Can you work these out from the model? Positions are in its coordinate system, mm. Face numbers are marked on the shaded views. A direction names the side the tool comes from. Round coordinates to 2 decimals unless told otherwise and drop trailing zeros. Loops run counter-clockwise (first coordinate to the right, second up) from the corner with the lowest first, then second, coordinate; pieces in that order, holes last. Notation, with made-up numbers: (-16.5, 27) -> (-3.5, 27) arc R22 ccw to (-3.5, 37) -> close; hole circle Ø8 at (9, 66). An arc over 180 degrees is marked (long way). Write each question's results on one line, items separated by ' | '.
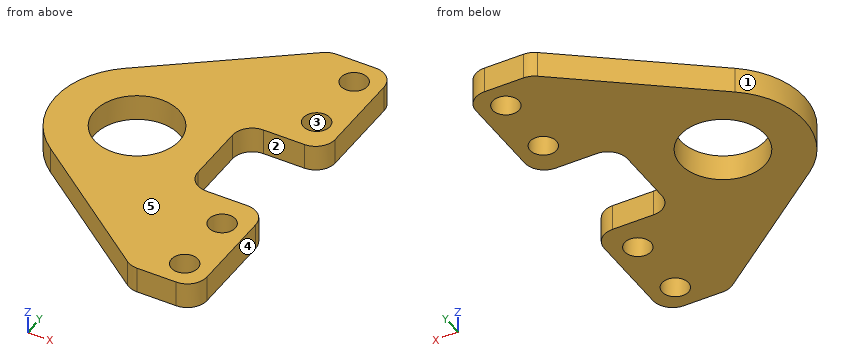
from build123d import *

# Parameters (mm, degrees)
SKETCH_1_R          = 6.5
SKETCH_1_R_2        = 2.025
EXTRUDE_1_DEPTH     = 2
SKETCH_2_W          = 12.3
SKETCH_2_H          = 15.2
CUT_EXTRUDE_1_DEPTH = 10
FILLET_1_R          = 3


with BuildPart() as part:
    # 草图1 → 凸台-拉伸1 (new, symmetric)
    with BuildSketch(Plane.XY):
        with BuildLine():
            Line((-7.572670512, 9.945082268), (14.3, 26.6))
            Line((14.3, 26.6), (24.3, 26.6))
            Line((24.3, 26.6), (24.3, -26.6))
            Line((24.3, -26.6), (14.3, -26.6))
            Line((14.3, -26.6), (-7.572670512, -9.945082268))
            ThreePointArc((-7.572670512, -9.945082268), (-12.5, 0), (-7.572670512, 9.945082268))
        make_face()
        Circle(SKETCH_1_R, mode=Mode.SUBTRACT)
        with Locations((20.3, 22.6)):
            Circle(SKETCH_1_R_2, mode=Mode.SUBTRACT)
        with Locations((20.3, 12.6)):
            Circle(SKETCH_1_R_2, mode=Mode.SUBTRACT)
        with Locations((20.3, -12.6)):
            Circle(SKETCH_1_R_2, mode=Mode.SUBTRACT)
        with Locations((20.3, -22.6)):
            Circle(SKETCH_1_R_2, mode=Mode.SUBTRACT)
    extrude(amount=EXTRUDE_1_DEPTH, both=True)

    # 草图2 → 切除-拉伸1 (cut)
    with BuildSketch(Plane.XY.offset(2)):
        with Locations((18.15, 0)):
            Rectangle(SKETCH_2_W, SKETCH_2_H)
    extrude(amount=-CUT_EXTRUDE_1_DEPTH, mode=Mode.SUBTRACT)

    # 圆角1
    fillet_1_edges = [part.edges().sort_by_distance(p)[0] for p in [
        (24.3, -26.6, 0),
        (14.3, -26.6, 0),
        (14.3, 26.6, 0),
        (24.3, 26.6, 0),
        (24.3, 7.6, 0),
        (24.3, -7.6, 0),
        (12, -7.6, 0),
        (12, 7.6, 0),
    ]]
    fillet(fillet_1_edges, radius=FILLET_1_R)


solid = part.part
1. If we section it at A-A (y = 0): List the corners of the cut face in (x, z) for me, then the cut area to 3 significant figures.
Final values:
outline: (-12.5, -2) -> (-6.5, -2) -> (-6.5, 2) -> (-12.5, 2) -> close; (6.5, -2) -> (12, -2) -> (12, 2) -> (6.5, 2) -> close | area: 46.0 mm2
2. Please list where these lines run through material, in increasing order: line 1 (Y direction, x = 20.3, z = 0.2) (3 decimals); line 2 (X direction, y = -4, z = 1); line 3 (X direction, y = 3.5, z = -1.8). Write a range as from..to.
Final values:
line 1: -26.6..-24.625, -20.575..-14.625, -10.575..-7.6, 7.6..10.575, 14.625..20.575, 24.625..26.6 | line 2: -11.84..-5.12, 5.12..12 | line 3: -12..-5.48, 5.48..12
3. If we section it at D-D (x = 20.3): List the corners of the cut face in (y, z) for me (3 decimals), then the cut area to 3 significant figures.
Final values:
outline: (-26.6, -2) -> (-24.625, -2) -> (-24.625, 2) -> (-26.6, 2) -> close; (-20.575, -2) -> (-14.625, -2) -> (-14.625, 2) -> (-20.575, 2) -> close; (-10.575, -2) -> (-7.6, -2) -> (-7.6, 2) -> (-10.575, 2) -> close; (7.6, -2) -> (10.575, -2) -> (10.575, 2) -> (7.6, 2) -> close; (14.625, -2) -> (20.575, -2) -> (20.575, 2) -> (14.625, 2) -> close; (24.625, -2) -> (26.6, -2) -> (26.6, 2) -> (24.625, 2) -> close | area: 87.2 mm2
4. If we section it at C-C (x = 0): List the corners of the cut face in (y, z) for me, then the cut area to 3 significant figures.
Final values:
outline: (-15.71, -2) -> (-6.5, -2) -> (-6.5, 2) -> (-15.71, 2) -> close; (6.5, -2) -> (15.71, -2) -> (15.71, 2) -> (6.5, 2) -> close | area: 73.7 mm2
5. Will these pins go through, and if not, where does the flat tip stop? pin 1 (3.5 mm diameter, centred on x = 20.3, y = -22.6, fed in from +Z); pin 2 (2 mm diameter, centred on y = 13.5, z = 0, fed in from -X); pin 3 (2 mm diameter, centred on y = -0.5, z = 0, fed in from +X); pin 4 (1 mm diameter, centred on y = 10.5, z = 1, fed in from -X).
Final values:
pin 1: through | pin 2: x = -4.22 | pin 3: x = 12 | pin 4: x = -7.5
6. We'd pull the mould along X, two halves only. Please class the marked faces 3, 4 and 5: pulls with the +X half, pulls with the -X half, needs draft (parallel to the pull), parting line crosses it, or undercut.
Final values:
face 3: undercut | face 4: pulls with the +X half | face 5: needs draft
7. If we section it at B-B (z = 1.45): List the corners of the cut face in (x, y) for me (3 decimals), then the cut area to 3 significant figures.
Final values:
outline: (-7.573, -9.945) -> (13.495, -25.987) arc R3 ccw to (15.312, -26.6) -> (21.3, -26.6) arc R3 ccw to (24.3, -23.6) -> (24.3, -10.6) arc R3 ccw to (21.3, -7.6) -> (15, -7.6) arc R3 cw to (12, -4.6) -> (12, 4.6) arc R3 cw to (15, 7.6) -> (21.3, 7.6) arc R3 ccw to (24.3, 10.6) -> (24.3, 23.6) arc R3 ccw to (21.3, 26.6) -> (15.312, 26.6) arc R3 ccw to (13.495, 25.987) -> (-7.573, 9.945) arc R12.5 ccw to start; hole circle Ø13 at (0, 0); hole circle Ø4.05 at (20.3, -22.6); hole circle Ø4.05 at (20.3, -12.6); hole circle Ø4.05 at (20.3, 12.6); hole circle Ø4.05 at (20.3, 22.6) | area: 1,020 mm2
8. On a 3-axis mill with a long thin cutter (end or side, diameter ignored), from which of +Z, -Z, +X, -X, +Y, -Y can I reach the whole of each face in a straight line? I mean the marked faces 1 and 2. Say none if no direction works.
Final values:
face 1: +Z, -Z, -X | face 2: +Z, -Z, +X
